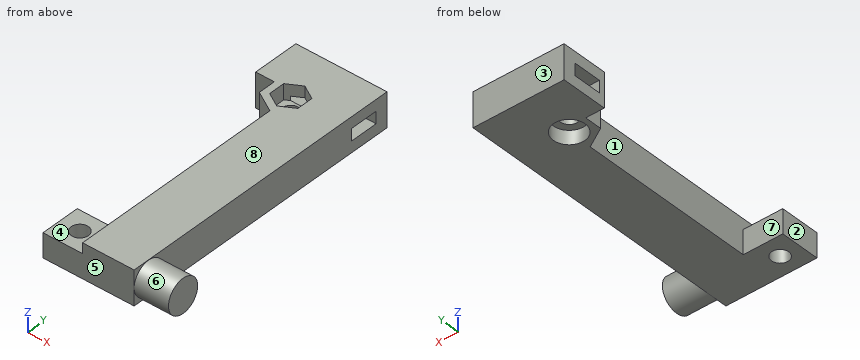
```python
from build123d import *

# Parameters (mm, degrees)
F0_W      = 15
F0_H      = 83
F1_DEPTH  = 10
F2_W      = 11.5
F2_H      = 11.5
F3_DEPTH  = 10
F4_W      = 11.5
F4_H      = 11.5
F5_DEPTH  = 10
F6_W      = 8.2
F6_H      = 3.5
F7_DEPTH  = 26.501
F9_DEPTH  = 10
F11_DEPTH = 4.5
F12_R     = 4.6
F13_DEPTH = 4
F14_R     = 2.5
F15_DEPTH = 1.5
F16_W     = 11.5
F16_H     = 11.5
F17_DEPTH = 3
F18_R     = 2.5
F19_DEPTH = 7
F20_R     = 4.9
F21_DEPTH = 10
F22_W     = 26.5
F22_H     = 2
F23_DEPTH = 10


with BuildPart() as f1:
    # F0 (on Top) → F1 (new body)
    with BuildSketch(Plane.XY):
        with Locations((-7.5, 41.5)):
            Rectangle(F0_W, F0_H)
    extrude(amount=F1_DEPTH)

    # F2 (on Top) → F3 (join, through all)
    with BuildSketch(Plane.XY):
        with Locations((-20.75, 5.75)):
            Rectangle(F2_W, F2_H)
    extrude(amount=F3_DEPTH)

    # F4 (on Top) → F5 (join, through all)
    with BuildSketch(Plane.XY):
        with Locations((-20.75, 77.25)):
            Rectangle(F4_W, F4_H)
    extrude(amount=F5_DEPTH)

    # F6 (on face) → F7 (cut, through all)
    with BuildSketch(Plane(origin=(-26.5, 0, 0), x_dir=(0, -1, 0), z_dir=(-1, 0, 0))):
        with Locations((-77.25, 5)):
            Rectangle(F6_W, F6_H)
    extrude(amount=-F7_DEPTH, mode=Mode.SUBTRACT)

    # F8 (on Top) → F9 (join, through all)
    with BuildSketch(Plane.XY):
        Polygon((-21.1, 66.478163), (-15, 62.956327), (-15, 71.5), (-21.1, 71.5), align=None)
    extrude(amount=F9_DEPTH)

    # F10 (on face) → F11 (cut)
    with BuildSketch(Plane.XY.offset(10)):
        Polygon((-19.1, 72.367136), (-19.1, 67.632864), (-15, 65.265728), (-10.9, 67.632864), (-10.9, 72.367136), (-15, 74.734272), align=None)
    extrude(amount=-F11_DEPTH, mode=Mode.SUBTRACT)

    # F12 (on face) → F13 (cut)
    with BuildSketch(Plane(origin=(0, 0, 0), x_dir=(1, 0, 0), z_dir=(0, 0, -1))):
        with Locations((-15, -70)):
            Circle(F12_R)
    extrude(amount=-F13_DEPTH, mode=Mode.SUBTRACT)

    # F14 (on face) → F15 (cut, through all)
    with BuildSketch(Plane(origin=(0, 0, 4), x_dir=(1, 0, 0), z_dir=(0, 0, -1))):
        with Locations((-15, -70)):
            Circle(F14_R)
    extrude(amount=-F15_DEPTH, mode=Mode.SUBTRACT)

    # F16 (on face) → F17 (cut)
    with BuildSketch(Plane.XY.offset(10)):
        with Locations((-20.75, 5.75)):
            Rectangle(F16_W, F16_H)
    extrude(amount=-F17_DEPTH, mode=Mode.SUBTRACT)

    # F18 (on face) → F19 (cut, through all)
    with BuildSketch(Plane.XY.offset(7)):
        with Locations((-20.75, 5.75)):
            Circle(F18_R)
    extrude(amount=-F19_DEPTH, mode=Mode.SUBTRACT)

    # F20 (on face) → F21 (join)
    with BuildSketch(Plane.YZ):
        with Locations((4.9, 5)):
            Circle(F20_R)
    extrude(amount=F21_DEPTH)

    # F22 (on Top) → F23 (join, through all)
    with BuildSketch(Plane.XY):
        with Locations((-13.25, 84)):
            Rectangle(F22_W, F22_H)
    extrude(amount=F23_DEPTH)


solid = f1.part
```
Design review of the part built by this model. Coordinates are the model's own, in mm. Face numbers are marked on the shaded views. A direction names the side the tool comes from. Give positions to 0.01 mm unless a question says otherwise; leave off trailing zeros. Loops run counter-clockwise (first coordinate to the right, second up) from the corner with the lowest first, then second, coordinate; pieces in that order, holes last. Notation, with made-up numbers: (-2, 72.25) -> (52, 72.25) arc R27 ccw to (52, 101.25) -> close; hole circle Ø6 at (29, 62). An arc over 180 degrees is marked (long way). One line per item, written item: value.
Q1. Draft analysis for pull direction Y (two halves, no side actions). For the marked faces 1, 2 and 3, state which applies: pulls with the +Y half, pulls with the -Y half, needs draft (parallel to the pull), parting line crosses it, or undercut.
Numbers:
face 1: undercut
face 2: needs draft
face 3: pulls with the +Y half
Q2. Machinability: for the marked faces 4, 5, 6, 7 and 8, which of the approach directions +Z, -Z, +X, -X, +Y, -Y give a long, thin tool a straight path to every point of the face, cutting with its end or side? Answer none if there is none.
Numbers:
face 4: +Z, -X, -Y
face 5: +Z, -Z, +X, -X, -Y
face 6: +X
face 7: +Z, -Z, -X
face 8: +Z, +X, -X, +Y, -Y
Q3. For L1, parallel to X at y = 70, z = 2.45; L2, parallel to Y at x = -2.5, z = 5.5; L3, parallel to X at y = 70, z = 4.5, list the stretches that pass through material, from the lowest coordinate up.
Numbers:
L1: x = -21.1 to -19.6, -10.4 to 0
L2: y = 0 to 73.15, 81.35 to 85
L3: x = -21.1 to -17.5, -12.5 to 0
Q4. We need section A-A on y = 76. Give the boundary of the cut face in (x, z), and give its area (3 significant figures).
Numbers:
outline: (-26.5, 0) -> (0, 0) -> (0, 3.25) -> (-26.5, 3.25) -> close; (-26.5, 6.75) -> (0, 6.75) -> (0, 10) -> (-26.5, 10) -> close
area: 172 mm^2
Q5. We need section D-D on x = 5. Give the boundary of the cut face in (y, z).
Numbers:
outline: circle Ø9.8 at (4.9, 5)
Q6. We need section C-C on z = 9. Give the boundary of the cut face in (x, y).
Numbers:
outline: (-26.5, 71.5) -> (-21.1, 71.5) -> (-21.1, 66.48) -> (-15, 62.96) -> (-15, 0) -> (0, 0) -> (0, 2.07) -> (10, 2.07) -> (10, 7.73) -> (0, 7.73) -> (0, 85) -> (-26.5, 85) -> close; hole (-19.1, 67.63) -> (-15, 65.27) -> (-10.9, 67.63) -> (-10.9, 72.37) -> (-15, 74.73) -> (-19.1, 72.37) -> close
Q7. We need section B-B on x = -5. Give the boundary of the cut face in (y, z), and give its area (3 significant figures).
Numbers:
outline: (0, 0) -> (85, 0) -> (85, 10) -> (0, 10) -> close; hole (73.15, 3.25) -> (81.35, 3.25) -> (81.35, 6.75) -> (73.15, 6.75) -> close
area: 821 mm^2
Q8. For pin 1 Ø6 at (y, z) = (60, 6) entering from -X; pin 2 Ø3 at (x, z) = (-8.5, 4.5) entering from -Y; pin 3 Ø3 at (y, z) = (20.5, 2.5) entering from -X; pin 4 Ø3.5 at (y, z) = (69.5, 9) entering from -X, all flat-tipped, find the tip position at first contact; note any pin that passes through.
Numbers:
pin 1: stops at x = -15.08
pin 2: stops at y = 0
pin 3: stops at x = -15
pin 4: stops at x = -21.1
